from build123d import *

# Parameters (mm, degrees)
F2_W     = 10
F2_H     = 3
F3_DEPTH = 12.5
F5_R     = 2
F6_DEPTH = 25
F8_DEPTH = 12.5


with BuildPart() as f1:
    # F0 (on Top) → F1 (revolve)
    with BuildSketch(Plane.XY):
        with BuildLine():
            ThreePointArc((0, -2.5), (-2.5, 0), (0, 2.5))
            Line((0, 2.5), (0, 4))
            ThreePointArc((0, 4), (-4, 0), (0, -4))
            Line((0, -4), (0, -2.5))
        make_face()
    revolve(axis=Axis((0, 0, 0), (0, -1, 0)))

    # F2 (on Top) → F3 (intersect, symmetric)
    with BuildSketch(Plane.XY):
        Rectangle(F2_W, F2_H)
    extrude(amount=F3_DEPTH, both=True, mode=Mode.INTERSECT)

    # F5 (on offset) → F6 (join)
    with BuildSketch(Plane.YZ.offset(-3)):
        Circle(F5_R)
    extrude(amount=-F6_DEPTH)

    # F7 (on Top) → F8 (cut, symmetric)
    with BuildSketch(Plane.XY):
        Polygon((-5, 2), (-3, 1.5), (3.708099, 1.5), (9, 1.5), (9, -1.5), (3.708099, -1.5), (-3, -1.5), (-5, -2), (-3, -2), (10, -2), (10, 2), (-3, 2), align=None)
    extrude(amount=F8_DEPTH, both=True, mode=Mode.SUBTRACT)


solid = f1.part
Read the model definition and answer for the solid it produces. Units are mm, in the model's axes. A direction names the side the tool comes from. Coordinates: 2 decimals unless noted, no trailing zeros. Write each loop counter-clockwise with the first axis right and the second up, starting at its lowest first coordinate (ties: lowest second). Pieces come first, ordered by that corner, then holes. Notation, with made-up numbers: M 53,4.25 L 72,4.25 A8 ccw 72,12.25 Z; hole C -0.5,-23 d7. An arc over 180 degrees is marked long. Use a Markdown table: item, result.
Q1. Which of the six approach directions +Z, -Z, +X, -X, +Y, -Y give full straight-line access (tool end or side, diameter ignored) to faces 1 (the face through (-3.8, 1.7, 0)), 2 (the face through (-15, -2, 0))?
Answer block:
| item | result |
|---|---|
| face 1 | +Z, -Z, +X, +Y |
| face 2 | -X |
Q2. The part is cut by section B-B, the plane x = 0. Write down the section's boundary in (y, z).
Answer block:
| item | result |
|---|---|
| outline | M -1.5,-3.71 A4 ccw 1.5,-3.71 L 1.5,-2 A2.5 cw -1.5,-2 Z; M -1.5,2 A2.5 cw 1.5,2 L 1.5,3.71 A4 ccw -1.5,3.71 Z |
Q3. Straight lines are drawn through the part: L1, parallel to X at y = -0.9, z = 0; L2, parallel to X at y = -1.4, z = 0.5; L3, parallel to Z at x = -23.5, y = -0.05. For each, find the intervals that lie inside material, in ascending order. Write a range as [from, to].
Answer block:
| item | result |
|---|---|
| L1 | x = [-28, -2.33], [2.33, 3.9] |
| L2 | x = [-28, -2.01], [2.01, 3.71] |
| L3 | z = [-2, 2] |
Q4. Each of these flat-tipped pins is pushed along its axis until it touches: pin 1 Ø2 at (y, z) = (-0.5, 1.5) entering from +X; pin 2 Ø2 at (x, z) = (-1, -1.5) entering from +Y. Where does it stop, or does it pass through?
Answer block:
| item | result |
|---|---|
| pin 1 | stops at x = 3.96 |
| pin 2 | stops at y = 1.5 |
Q5. The part is cut by section C-C, the plane y = -0.75. Write down the section's boundary in (x, z), then the cut area to 3 significant figures.
Answer block:
| item | result |
|---|---|
| outline | M -28,-1.85 L -3.46,-1.85 A3.93 ccw long -3.46,1.85 L -28,1.85 Z; hole C 0,0 d4.77 |
| area | 120 mm2 |
Q6. The part is cut by section A-A, the plane z = 0. Write down the section's boundary in (x, y).
Answer block:
| item | result |
|---|---|
| outline | M -28,-2 L -5,-2 L -3,-1.5 L -2,-1.5 A2.5 cw -2,1.5 L -3,1.5 L -5,2 L -28,2 Z; M 2,-1.5 L 3.71,-1.5 A4 ccw 3.71,1.5 L 2,1.5 A2.5 cw Z |
Q7. The part is cut by section D-D, the plane x = -7.5. Write down the section's boundary in (y, z), then the cut area to 3 significant figures.
Answer block:
| item | result |
|---|---|
| outline | C 0,0 d4 |
| area | 12.6 mm2 |
